```python
from build123d import *

# Parameters (mm, degrees)
SKETCH_1_R      = 1.5
EXTRUDE_1_DEPTH = 3
SKETCH_2_W      = 23.5
SKETCH_2_H      = 11
SKETCH_2_R      = 1.5
SKETCH_2_W_2    = 1
SKETCH_2_W_3    = 15
EXTRUDE_2_DEPTH = 7
FILLET_2_R      = 3
EXTRUDE_3_DEPTH = 8
FILLET_3_R      = 3
FILLET_4_R      = 3


with BuildPart() as part:
    # 草图1 → 凸台-拉伸1 (new body)
    with BuildSketch(Plane(origin=(0, 0, 0), x_dir=(1, 0, 0), z_dir=(0, 1, 0))):
        Polygon((-23.5, 19), (-23.5, -19), (1, -19), (1, -7), (13, -7), (13, -19), (23.5, -19), (23.5, 19), align=None)
        with Locations(Location((-19.5, -14, 0), (0, 0, 270))):
            Circle(SKETCH_1_R, mode=Mode.SUBTRACT)
        with Locations(Location((19.5, -14, 0), (0, 0, 270))):
            Circle(SKETCH_1_R, mode=Mode.SUBTRACT)
        with Locations(Location((-19.5, 14, 0), (0, 0, 270))):
            Circle(SKETCH_1_R, mode=Mode.SUBTRACT)
        with Locations(Location((19.5, 14, 0), (0, 0, 270))):
            Circle(SKETCH_1_R, mode=Mode.SUBTRACT)
    extrude(amount=EXTRUDE_1_DEPTH)

    # 草图2 → 凸台-拉伸2 (add)
    # profile 1 of 3: a face of its own
    with BuildSketch(Plane.XY.offset(19)):
        with Locations((-11.75, 5.5)):
            Rectangle(SKETCH_2_W, SKETCH_2_H)
        with Locations((-20, 7)):
            Circle(SKETCH_2_R, mode=Mode.SUBTRACT)
        with Locations((-12, 7)):
            Circle(SKETCH_2_R, mode=Mode.SUBTRACT)
    # profile 2 of 3: a face of its own
    with BuildSketch(Plane.XY.offset(19)):
        with Locations((0.5, 5.5)):
            Rectangle(SKETCH_2_W_2, SKETCH_2_H)
    # profile 3 of 3: a face of its own
    with BuildSketch(Plane.XY.offset(19)):
        with Locations((16, 5.5)):
            Rectangle(SKETCH_2_W_3, SKETCH_2_H)
        with Locations((12, 7)):
            Circle(SKETCH_2_R, mode=Mode.SUBTRACT)
        with Locations((20, 7)):
            Circle(SKETCH_2_R, mode=Mode.SUBTRACT)
    extrude(amount=EXTRUDE_2_DEPTH)

    # 圆角2
    fillet_2_edges = [part.edges().sort_by_distance(p)[0] for p in [
        (-23.5, 1.5, -19),
        (23.5, 1.5, -19),
    ]]
    fillet(fillet_2_edges, radius=FILLET_2_R)

    # 草图3 → 凸台-拉伸3 (add)
    with BuildSketch(Plane(origin=(1, 0, 0), x_dir=(0, 0, -1), z_dir=(1, 0, 0))):
        Polygon((-19, 11), (-19, 8), (-4, 3), (5, 3), align=None)
    extrude(amount=-EXTRUDE_3_DEPTH)

    # 圆角3
    fillet_3_edges = [part.edges().sort_by_distance(p)[0] for p in [
        (13, 1.5, 19),
    ]]
    fillet(fillet_3_edges, radius=FILLET_3_R)

    # 圆角4
    fillet_4_edges = [part.edges().sort_by_distance(p)[0] for p in [
        (-23.5, 11, 22.5),
        (23.5, 11, 22.5),
        (8.5, 11, 22.5),
    ]]
    fillet(fillet_4_edges, radius=FILLET_4_R)


solid = part.part
```
Geometry check sheet. Reference: the model listing, model coordinates, mm. A direction names the side the tool comes from. Give positions to 0.01 mm unless a question says otherwise; leave off trailing zeros. Order: outer loops, then holes, each group sorted by start corner. A loop starts at its lowest first (then second) coordinate and runs counter-clockwise, first axis right, second up.
1. Access from +Z, -Z, +X, -X, +Y, -Y to the whole of each face (thin tool, end or side, straight path). Record for faces 5 (the face through (7, 1, 7)), 6 (the face through (8.5, 4, 22)), 7 (the face through (9.4, 10.14, 22.55)).
2. Gauge pin test, flat ends, axial feed: pin 1 Ø6 at (x, y) = (-15.5, 7) entering from -Z; pin 2 Ø4 at (y, z) = (6, 7) entering from -X; pin 3 Ø5 at (x, z) = (19.5, 14) entering from +Y; pin 4 Ø2.5 at (x, y) = (-12, 7) entering from +Z. Record the tip position at first contact, or that the pin passes through.
3. Section check D-D, the plane x = -19.5. Enter the section's corners in (y, z), and give its area (3 significant figures).
4. Section check A-A, the plane z = -14. Enter the section's corners in (x, y).
5. Section check C-C, the plane y = 1.25. Enter the section's corners in (x, z).
6. Release check for a two-part mould opening along Z. For faces 1 (the face through (-11, 4, 26)), 2 (the face through (12.14, 1.52, 18.1)), 3 (the face through (-18.49, 1.48, 12.89)), 4 (the face through (1, 7, 14)) record: pulls with the +Z half, pulls with the -Z half, needs draft (parallel to the pull), parting line crosses it, or undercut.
7. Thickness scan on L1, parallel to X at y = 2.1, z = -14; L2, parallel to Y at x = -12, z = 22; L3, parallel to X at y = 2, z = 9. Record the ranges inside material, lowest first.
8. Section check B-B, the plane y = 7. Enter the section's corners in (x, z), and give its area (4 significant figures).
Values follow:
1. face 5: +Y, -Y
1. face 6: +Z, +Y, -Y
1. face 7: +Z, -Z, +Y
2. pin 1: stops at z = 19
2. pin 2: stops at x = -7
2. pin 3: stops at y = 3
2. pin 4: passes through
3. outline: (0, -19) - (3, -19) - (3, -15.5) - (0, -15.5) - close; (0, -12.5) - (3, -12.5) - (3, 12.5) - (0, 12.5) - close; (0, 15.5) - (3, 15.5) - (3, 19) - (5.59, 19) - (5.59, 26) - (0, 26) - close; (8.41, 19) - (11, 19) - (11, 26) - (8.41, 26) - close
3. area: 153 mm2
4. outline: (-23.5, 0) - (-21, 0) - (-21, 3) - (-23.5, 3) - close; (-18, 0) - (18, 0) - (18, 3) - (-18, 3) - close; (21, 0) - (23.5, 0) - (23.5, 3) - (21, 3) - close
5. outline: (-23.5, -16) arc R3 ccw to (-20.5, -19) - (20.5, -19) arc R3 ccw to (23.5, -16) - (23.5, 26) - (8.5, 26) - (8.5, 19) - (10, 19) arc R3 cw to (13, 16) - (13, 7) - (1, 7) - (1, 26) - (-23.5, 26) - close; hole circle Ø3 at (-19.5, -14); hole circle Ø3 at (-19.5, 14); hole circle Ø3 at (19.5, -14); hole circle Ø3 at (19.5, 14)
6. face 1: pulls with the +Z half
6. face 2: undercut
6. face 3: undercut
6. face 4: needs draft
7. L1: x = -23.5 to -21, -18 to 18, 21 to 23.5
7. L2: y = 0 to 5.5, 8.5 to 11
7. L3: x = -23.5 to 1, 13 to 23.5
8. outline: (-23.5, 19) - (-21.5, 19) - (-21.5, 26) - (-23.5, 26) - close; (-18.5, 19) - (-13.5, 19) - (-13.5, 26) - (-18.5, 26) - close; (-10.5, 19) - (1, 19) - (1, 26) - (-10.5, 26) - close; (-7, 7) - (1, 7) - (1, 16) - (-7, 16) - close; (8.5, 19) - (10.5, 19) - (10.5, 26) - (8.5, 26) - close; (13.5, 19) - (18.5, 19) - (18.5, 26) - (13.5, 26) - close; (21.5, 19) - (23.5, 19) - (23.5, 26) - (21.5, 26) - close
8. area: 264.5 mm2
